Can you work these out from the model? Positions are in its coordinate system, mm. Face numbers are marked on the shaded views. Give positions to 0.01 mm unless a question says otherwise; leave off trailing zeros. Loops run counter-clockwise (first coordinate to the right, second up) from the corner with the lowest first, then second, coordinate; pieces in that order, holes last. Notation, with made-up numbers: M 74,70 L 100,70 A5 ccw 100,75 Z; hole C 31.5,76 d7. An arc over 180 degrees is marked long. Put each result on its own line as item: value. Start each with the question number.
1) Please list where these lines run through material, in increasing order: line 1 along Z through (x, y) = (17, 11.75); line 2 along X through (y, z) = (7, 4); line 3 along Y through (x, z) = (25, 22.5). Write a range as from..to.
2) Imagine slicing it at B-B (y = 5). Write out the boundary of the cut face in (x, z).
3) Imagine slicing it at A-A (z = 27). Write out the boundary of the cut face in (x, y).
4) If we mould it in two halves opening along Y, with no side actions, what happens to the marked faces 1, 2, 3 and 4? For each: +Y half, -Y half, draft (parallel to the pull), parting line (faces both ways), or undercut.
5) Imagine slicing it at C-C (x = 27). Write out the boundary of the cut face in (y, z).
6) Imagine slicing it at D-D (z = 21). Write out the boundary of the cut face in (x, y).
7) For P1, Ø12, axis at x = 24, z = 17.5, coming from the +Y side; P2, Ø6, axis at x = 36, y = 16.5, coming from the +Z side; P3, Ø4, axis at y = 8, z = 5.5, coming from the +X side; P4, Ø4, axis at y = 3, z = 14, coming from the -X side, each with a flat end and sliding along its axis, tell me the tip position at first contact or that it passes through.
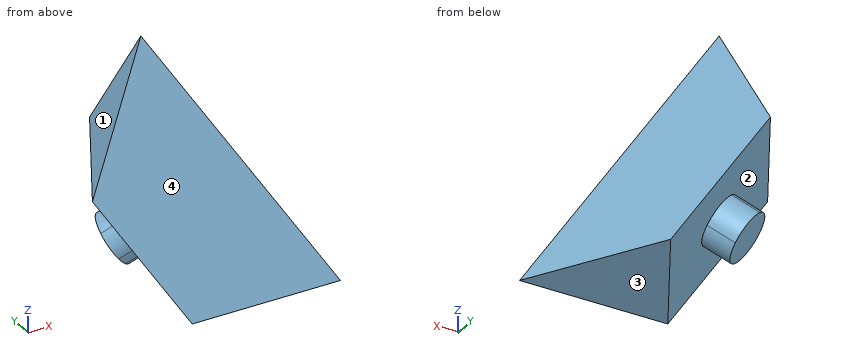
from build123d import *

# Parameters (mm, degrees)
F7_DEPTH = 4


with BuildPart() as f3:
    # F0 (on Top) → F3 section 0
    with BuildSketch(Plane.XY, mode=Mode.PRIVATE) as f3_s0:
        Polygon((20, 34.6410161514), (0, 0), (40, 0), align=None)
    loft([f3_s0.sketch, Vertex(20, 11.5470053838, 32.6598632371)])

    # F5: sweep along a path in F5_path
    with BuildLine(Plane(origin=(0, 0, 0), x_dir=(-0.5, -0.8660254038, 0), z_dir=(0.8660254038, -0.5, 0))) as f5_path:
        Line((0, 0), (-40, 0))
    # F4 (on face) → F5 (sweep, cut)
    with BuildSketch(Plane(origin=(26.6666666667, 15.3960071784, 10.886621079), x_dir=(-0.4364357805, 0.8819171037, -0.1781741613), z_dir=(0.8164965809, 0.4714045208, 0.3333333333))):
        Polygon((2.1821789024, -11.3389341903), (21.8217890236, -7.5592894602), (8.7287156094, 7.5592894602), align=None)
    sweep(path=f5_path.line, mode=Mode.SUBTRACT)

    # F6 (on face) → F7 (join)
    with BuildSketch(Plane(origin=(10, -5.7735026919, 8.1649658093), x_dir=(-0.316227766, -0.9128709292, -0.2581988897), z_dir=(-0.7071067812, 0.4082482905, -0.5773502692))):
        with BuildLine():
            ThreePointArc((-17.4084183768, -3.1940601518), (-20.0804631421, -3.0041637772), (-22.1041611295, -4.7593077361))
            Line((-22.1041611295, -4.7593077361), (-18.973665961, -6.3245553203))
            Line((-18.973665961, -6.3245553203), (-17.4084183768, -3.1940601518))
        make_face()
        with BuildLine():
            Line((-17.4084183768, -3.1940601518), (-18.973665961, -6.3245553203))
            Line((-18.973665961, -6.3245553203), (-15.8431707925, -7.8898029046))
            ThreePointArc((-15.8431707925, -7.8898029046), (-15.5672944979, -7.1286905423), (-15.473665961, -6.3245553203))
            ThreePointArc((-15.473665961, -6.3245553203), (-15.9963881318, -4.4844964279), (-17.4084183768, -3.1940601518))
        make_face()
        with BuildLine():
            Line((-18.973665961, -6.3245553203), (-22.1041611295, -4.7593077361))
            ThreePointArc((-22.1041611295, -4.7593077361), (-22.2940575042, -7.4313525014), (-20.5389135453, -9.4550504888))
            Line((-20.5389135453, -9.4550504888), (-18.973665961, -6.3245553203))
        make_face()
        with BuildLine():
            Line((-15.8431707925, -7.8898029046), (-18.973665961, -6.3245553203))
            Line((-18.973665961, -6.3245553203), (-20.5389135453, -9.4550504888))
            ThreePointArc((-20.5389135453, -9.4550504888), (-17.86686878, -9.6449468635), (-15.8431707925, -7.8898029046))
        make_face()
    extrude(amount=F7_DEPTH)


solid = f3.part
Recorded:
1. line 1: 5.05..10.22, 11.98..25.02
1. line 2: 20.78..34.33
1. line 3: 7.95..10.07
2. outline: M 11.34,14.14 L 22.89,0 L 37.11,0 L 31.34,14.14 Z
3. outline: M 16.53,9.55 L 23.47,9.55 L 20,15.55 Z
4. face 1: +Y half
4. face 2: undercut
4. face 3: draft
4. face 4: -Y half
5. outline: M 0,0 L 12.12,0 L 19.05,4.9 L 7.51,21.23 Z
6. outline: M 12.86,7.42 L 27.14,7.42 L 20,19.79 Z
7. P1: y = 23.09
7. P2: through
7. P3: x = 34.55
7. P4: x = 11.35
